Can you work these out from the model? Positions are in its coordinate system, mm. Face numbers are marked on the shaded views. Round coordinates to 2 decimals unless told otherwise and drop trailing zeros. Order: outer loops, then holes, each group sorted by start corner. A loop starts at its lowest first (then second) coordinate and runs counter-clockwise, first axis right, second up.
Q1. If we section it at A-A (z = 36): Please give me the cut outline in (x, y), plus the area to 3 significant figures.
Q2. If we section it at C-C (x = 2.5): Please give me the cut outline in (y, z), plus the area to 3 significant figures.
Q3. We'd pull the mould along X, two halves only. Please class the marked faces 1, 2 and 3: pulls with the +X half, pulls with the -X half, needs draft (parallel to the pull), parting line crosses it, or undercut.
Q4. If we section it at B-B (y = 160.5): Please give me the cut outline in (x, z).
Q5. Will these pins go through, and if not, where does the flat tip stop? P1, Ø2, axis at x = -131.5, z = 303, coming from the +Y side; P2, Ø1, axis at x = -46, z = 163, coming from the +Y side; P3, Ø5, axis at x = -172.5, z = 263.5, coming from the -Y side.
Q6. If we section it at D-D (z = 129): Please give me the cut outline in (x, y), plus the area to 3 significant figures.
Q7. If I drill on line 1 (X direction, y = 96.5, z = 33.5); line 2 (Y direction, x = 11, z = 33); line 3 (Y direction, x = 35, z = 335.5), over which ranges is the centre line in solid material (lowest first)?
from build123d import *

# Parameters (mm, degrees)
F1_DEPTH = 400
F3_DEPTH = 550
F4_DEPTH = 330


with BuildPart() as f1:
    # F0 (on Top) → F1 (new body)
    with BuildSketch(Plane.XY):
        with BuildLine():
            Line((214.4711060817, 211.0624126145), (-213.2998602418, 211.0624126145))
            ThreePointArc((-213.2998602418, 211.0624126145), (-241.0972159396, 198.6720372021), (-249.9143754115, 169.5434930316))
            Line((-249.9143754115, 169.5434930316), (-249.9143754115, -158.3375933319))
            ThreePointArc((-249.9143754115, -158.3375933319), (-239.1857706386, -184.2264108639), (-213.289735862, -194.9375833684))
            Line((-213.289735862, -194.9375833684), (214.510264138, -194.6495638067))
            ThreePointArc((214.510264138, -194.6495638067), (240.3744404519, -183.9209673287), (251.0856212514, -158.0495737702))
            Line((251.0856212514, -158.0495737702), (251.0856212514, 169.5434930316))
            ThreePointArc((251.0856212514, 169.5434930316), (242.2684617794, 198.6720372021), (214.4711060817, 211.0624126145))
        make_face()
        with BuildLine():
            ThreePointArc((-246.9143770801, 169.7504262298), (-238.9080461949, 196.6185567775), (-213.3143770801, 208.0624142831))
            Line((-213.3143770801, 208.0624142831), (214.4856229199, 208.0624142831))
            ThreePointArc((214.4856229199, 208.0624142831), (240.0792920347, 196.6185567775), (248.0856229199, 169.7504262298))
            Line((248.0856229199, 169.7504262298), (248.0856229199, -158.0495737702))
            ThreePointArc((248.0856229199, -158.0495737702), (238.2524073114, -181.8003623821), (214.5082443671, -191.6495661551))
            Line((214.5082443671, -191.6495661551), (-213.2917556329, -191.9375857169))
            ThreePointArc((-213.2917556329, -191.9375857169), (-237.065165692, -182.1043777234), (-246.9143770801, -158.3375933319))
            Line((-246.9143770801, -158.3375933319), (-246.9143770801, 169.7504262298))
        make_face(mode=Mode.SUBTRACT)
    extrude(amount=F1_DEPTH)

    # F2 (on face) → F3 (cut)
    with BuildSketch(Plane.YZ.offset(251.0856212514)):
        with BuildLine():
            Line((169.5434930316, 400), (-134.6142441034, 400))
            Line((-134.6142441034, 400), (-75.4682049155, 152.0536094904))
            ThreePointArc((-75.4682049155, 152.0536094904), (-41.2013099843, 95.6971256436), (19.5434930316, 70))
            Line((19.5434930316, 70), (169.5434930316, 70))
            Line((169.5434930316, 70), (169.5434930316, 400))
        make_face()
    extrude(amount=-F3_DEPTH, mode=Mode.SUBTRACT)

    # F4 (cut): a face of the model
    f4_faces = [f1.faces().sort_by_distance(p)[0] for p in [
        (241.8909190901, 198.3390915797, 400),
    ]]
    extrude(f4_faces, amount=-F4_DEPTH, mode=Mode.SUBTRACT)


solid = f1.part
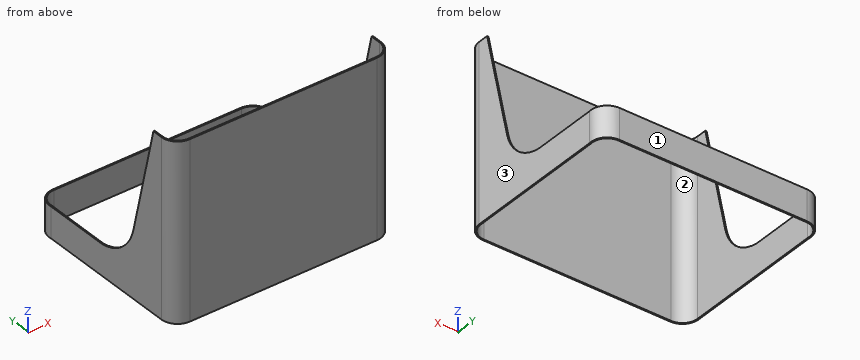
Solution:
1. outline: (-249.91, -158.34) arc R36.6 ccw to (-213.29, -194.94) - (214.51, -194.65) arc R36.6 ccw to (251.09, -158.05) - (251.09, 169.54) arc R36.6 ccw to (214.47, 211.06) - (-213.3, 211.06) arc R36.6 ccw to (-249.91, 169.54) - close; hole (-246.91, -158.34) arc R33.6 ccw to (-213.29, -191.94) - (214.51, -191.65) arc R33.6 ccw to (248.09, -158.05) - (248.09, 169.75) arc R33.6 ccw to (214.49, 208.06) - (-213.31, 208.06) arc R33.6 ccw to (-246.91, 169.75) - close
1. area: 5,230 mm2
2. outline: (-194.79, 0) - (-191.79, 0) - (-191.79, 400) - (-194.79, 400) - close; (208.06, 0) - (211.06, 0) - (211.06, 70) - (208.06, 70) - close
2. area: 1,410 mm2
3. face 1: needs draft
3. face 2: undercut
3. face 3: pulls with the +X half
4. outline: (-249.91, 0) - (-246.91, 0) - (-246.91, 70) - (-249.91, 70) - close; (248.09, 0) - (251.09, 0) - (251.09, 70) - (248.09, 70) - close
5. P1: stops at y = -191.88
5. P2: stops at y = -191.82
5. P3: stops at y = -194.91
6. outline: (-249.91, -158.34) arc R36.6 ccw to (-213.29, -194.94) - (214.51, -194.65) arc R36.6 ccw to (251.09, -158.05) - (251.09, -67.09) - (248.09, -67.09) - (248.09, -158.05) arc R33.6 cw to (214.51, -191.65) - (-213.29, -191.94) arc R33.6 cw to (-246.91, -158.34) - (-246.91, -67.09) - (-249.91, -67.09) - close
6. area: 2,160 mm2
7. line 1: x = -249.91 to -246.91, 248.09 to 251.09
7. line 2: y = -194.79 to -191.79, 208.06 to 211.06
7. line 3: y = -194.77 to -191.77
